The listing builds one solid part. Answer for the finished solid, in the listing's coordinates (mm). Face numbers are marked on the shaded views. A direction names the side the tool comes from. Coordinates: 2 decimals unless noted, no trailing zeros. Write each loop counter-clockwise with the first axis right and the second up, starting at its lowest first coordinate (ties: lowest second). Pieces come first, ordered by that corner, then holes.
(1) The part is cut by section B-B on y = 50. Determine the outline of the cut face in (x, z), plus the area to 3 significant figures.
(2) The part is cut by section D-D on z = -15. Determine the outline of the cut face in (x, y), plus the area to 3 significant figures.
(3) The part is cut by section A-A on y = 15. Determine the outline of the cut face in (x, z), plus the area to 3 significant figures.
(4) Straight lines are drawn through the part: line 1 (Y direction, x = 58, z = -35); line 2 (Y direction, x = 57, z = -35); line 3 (X direction, y = 24, z = -66). For each, find the intervals that lie inside material, in ascending order.
(5) For a pull along X with two mould halves and no side action, classify the marked faces 3, 4 and 5 as +X half, -X half, draft (parallel to the pull), parting line (faces both ways), or undercut.
(6) Given P1, Ø12, axis at x = -17.5, z = -31, coming from the +Y side; P2, Ø3.5, axis at y = 25, z = -10, coming from the -X side; P3, Ø3.5, axis at y = 35, z = -55, coming from the +X side, each flat-ended and moving along its own axis, determine where each tip first touches the part or whether it passes through.
(7) The part is cut by section C-C on x = -42. Determine the outline of the cut face in (y, z), plus the area to 3 significant figures.
(8) Which of the six approach directions +Z, -Z, +X, -X, +Y, -Y give full straight-line access (tool end or side, diameter ignored) to the marked faces 1 and 2?
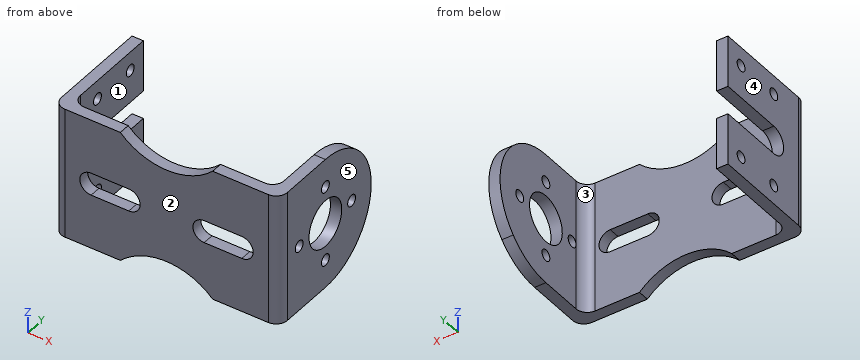
from build123d import *
from build123d.topology import SkipClean

# Parameters (mm, degrees)
BASEPLATEEXTRUDE_DEPTH = 70
FEATUREOP1_DEPTH       = 33
FEATUREOP2_DEPTH       = 6
SKETCH4_R              = 12.5
FEATUREOP3_DEPTH       = 16
SKETCH5_R              = 3
FEATUREOP4_DEPTH       = 16
SKETCH6_R              = 3
FEATUREOP5_DEPTH       = 16
FEATUREOP6_DEPTH       = 16


with BuildPart() as part:
    # Sketch1 → BasePlateExtrude (new body)
    with BuildSketch(Plane.XY):
        with BuildLine():
            Line((-54, 0), (54, 0))
            ThreePointArc((54, 0), (58.242640687, 1.757359313), (60, 6))
            Line((60, 6), (60, 60))
            Line((60, 60), (54, 60))
            Line((54, 60), (54, 12))
            ThreePointArc((54, 12), (52.242640687, 7.757359313), (48, 6))
            Line((48, 6), (-48, 6))
            ThreePointArc((-48, 6), (-52.242640687, 7.757359313), (-54, 12))
            Line((-54, 12), (-54, 60))
            Line((-54, 60), (-60, 60))
            Line((-60, 60), (-60, 6))
            ThreePointArc((-60, 6), (-58.242640687, 1.757359313), (-54, 0))
        make_face()
    extrude(amount=-BASEPLATEEXTRUDE_DEPTH)

    # Sketch2 → FeatureOp1 (cut)
    with BuildSketch(Plane(origin=(60, 0, 0), x_dir=(0, 0, -1), z_dir=(1, 0, 0))):
        with BuildLine():
            Line((0, 35), (0, 60))
            Line((0, 60), (10.505102572, 60))
            ThreePointArc((10.505102572, 60), (2.732978058, 48.558735008), (0, 35))
        make_face()
        with BuildLine():
            Line((70, 35), (70, 60))
            Line((70, 60), (59.494897428, 60))
            ThreePointArc((59.494897428, 60), (67.267021942, 48.558735008), (70, 35))
        make_face()
    extrude(amount=-FEATUREOP1_DEPTH, mode=Mode.SUBTRACT)

    # Sketch3 → FeatureOp2 (add)
    with SkipClean():  # the faces are left unmerged after this step: merging them gives an invalid solid
        with BuildSketch(Plane(origin=(60, 0, 0), x_dir=(0, 0, -1), z_dir=(1, 0, 0))):
            with BuildLine():
                Line((10.505102572, 60), (59.494897428, 60))
                ThreePointArc((59.494897428, 60), (35, 70), (10.505102572, 60))
            make_face()
        extrude(amount=-FEATUREOP2_DEPTH)

    # Sketch4 → FeatureOp3 (cut)
    with SkipClean():  # the faces are left unmerged after this step: merging them gives an invalid solid
        with BuildSketch(Plane(origin=(60, 0, 0), x_dir=(0, 0, -1), z_dir=(1, 0, 0))):
            with Locations((35, 35)):
                Circle(SKETCH4_R)
        extrude(amount=-FEATUREOP3_DEPTH, mode=Mode.SUBTRACT)

    # Sketch5 → FeatureOp4 (cut)
    with SkipClean():  # the faces are left unmerged after this step: merging them gives an invalid solid
        with BuildSketch(Plane(origin=(60, 0, 0), x_dir=(0, 0, -1), z_dir=(1, 0, 0))):
            with Locations((35, 55)):
                Circle(SKETCH5_R)
            with Locations((55, 35)):
                Circle(SKETCH5_R)
            with Locations((35, 15)):
                Circle(SKETCH5_R)
            with Locations((15, 35)):
                Circle(SKETCH5_R)
        extrude(amount=-FEATUREOP4_DEPTH, mode=Mode.SUBTRACT)

    # Sketch6 → FeatureOp5 (cut)
    with SkipClean():  # the faces are left unmerged after this step: merging them gives an invalid solid
        with BuildSketch(Plane.ZY.offset(60)):
            with Locations((-60, 50)):
                Circle(SKETCH6_R)
            with Locations((-60, 25)):
                Circle(SKETCH6_R)
            with Locations((-10, 50)):
                Circle(SKETCH6_R)
            with Locations((-10, 25)):
                Circle(SKETCH6_R)
            with BuildLine():
                Line((-42.5, 60), (-27.5, 60))
                Line((-27.5, 60), (-27.5, 25))
                ThreePointArc((-27.5, 25), (-35, 17.5), (-42.5, 25))
                Line((-42.5, 25), (-42.5, 60))
            make_face()
        extrude(amount=-FEATUREOP5_DEPTH, mode=Mode.SUBTRACT)

    # Sketch7 → FeatureOp6 (cut)
    with SkipClean():  # the faces are left unmerged after this step: merging them gives an invalid solid
        with BuildSketch(Plane(origin=(0, 6, 0), x_dir=(1, 0, 0), z_dir=(0, 1, 0))):
            with BuildLine():
                Line((-40, 41), (-20, 41))
                ThreePointArc((-20, 41), (-14, 35), (-20, 29))
                Line((-20, 29), (-40, 29))
                ThreePointArc((-40, 29), (-46, 35), (-40, 41))
            make_face()
            with BuildLine():
                Line((20, 29), (40, 29))
                ThreePointArc((40, 29), (46, 35), (40, 41))
                Line((40, 41), (20, 41))
                ThreePointArc((20, 41), (14, 35), (20, 29))
            make_face()
            with BuildLine():
                Line((-24.494897428, 0), (24.494897428, 0))
                ThreePointArc((24.494897428, 0), (0, 10), (-24.494897428, 0))
            make_face()
            with BuildLine():
                Line((-24.494897428, 70), (24.494897428, 70))
                ThreePointArc((24.494897428, 70), (0, 60), (-24.494897428, 70))
            make_face()
        extrude(amount=-FEATUREOP6_DEPTH, mode=Mode.SUBTRACT)


solid = part.part
Model answer:
1. outline: (-60, -70) - (-54, -70) - (-54, -63) - (-60, -63) - close; (-60, -57) - (-54, -57) - (-54, -42.5) - (-60, -42.5) - close; (-60, -27.5) - (-54, -27.5) - (-54, -13) - (-60, -13) - close; (-60, -7) - (-54, -7) - (-54, 0) - (-60, 0) - close; (54, -66.62) - (60, -66.62) - (60, -3.38) - (54, -3.38) - close
1. area: 637 mm2
2. outline: (-60, 6) arc R6 ccw to (-54, 0) - (54, 0) arc R6 ccw to (60, 6) - (60, 32) - (54, 32) - (54, 12) arc R6 cw to (48, 6) - (-48, 6) arc R6 cw to (-54, 12) - (-54, 60) - (-60, 60) - close; (54, 38) - (60, 38) - (60, 63.72) - (54, 63.72) - close
2. area: 1,350 mm2
3. outline: (-60, -70) - (-54, -70) - (-54, 0) - (-60, 0) - close; (54, -70) - (60, -70) - (60, -38) - (54, -38) - close; (54, -32) - (60, -32) - (60, 0) - (54, 0) - close
3. area: 804 mm2
4. line 1: y = 1.53 to 12, 18 to 22.5, 47.5 to 52, 58 to 70
4. line 2: y = 0.8 to 12, 18 to 22.5, 47.5 to 52, 58 to 70
4. line 3: x = -60 to -54, 54 to 60
5. face 3: undercut
5. face 4: -X half
5. face 5: +X half
6. P1: stops at y = 6
6. P2: stops at x = 54
6. P3: stops at x = -54
7. outline: (0, -70) - (6, -70) - (6, -40.66) - (0, -40.66) - close; (0, -29.34) - (6, -29.34) - (6, 0) - (0, 0) - close
7. area: 352 mm2
8. face 1: +Z, -Z, +Y
8. face 2: +Z, -Z, +X, -X, -Y
